```python
from build123d import *

# Parameters (mm, degrees)
ESBO_O1_W                = 36
ESBO_O1_H                = 55
RESSALTO_EXTRUS_O1_DEPTH = 75
ESBO_O2_W                = 34
ESBO_O2_H                = 30
CORTE_EXTRUS_O1_DEPTH    = 56
ESBO_O3_W                = 56
ESBO_O3_H                = 51
CORTE_EXTRUS_O2_DEPTH    = 57
ESBO_O5_R                = 5
CORTE_EXTRUS_O4_DEPTH    = 57
ESBO_O6_W                = 36
ESBO_O6_H                = 51
CORTE_EXTRUS_O5_DEPTH    = 16
ESBO_O4_R                = 5
CORTE_EXTRUS_O6_DEPTH    = 63


with BuildPart() as part:
    # Esboço1 → Ressalto-extrusão1 (new body)
    with BuildSketch(Plane.XY):
        Rectangle(ESBO_O1_W, ESBO_O1_H)
    extrude(amount=RESSALTO_EXTRUS_O1_DEPTH)

    # Esboço2 → Corte-extrusão1 (cut)
    with BuildSketch(Plane.XY.offset(75)):
        Rectangle(ESBO_O2_W, ESBO_O2_H)
    extrude(amount=-CORTE_EXTRUS_O1_DEPTH, mode=Mode.SUBTRACT)

    # Esboço3 → Corte-extrusão2 (cut)
    with BuildSketch(Plane.ZY.offset(18)):
        with Locations((47, 0)):
            Rectangle(ESBO_O3_W, ESBO_O3_H)
    extrude(amount=-CORTE_EXTRUS_O2_DEPTH, mode=Mode.SUBTRACT)

    # Esboço5 → Corte-extrusão4 (cut)
    with BuildSketch(Plane(origin=(0, 0, 0), x_dir=(-1, 0, 0), z_dir=(0, 0, -1))):
        Circle(ESBO_O5_R)
    extrude(amount=-CORTE_EXTRUS_O4_DEPTH, mode=Mode.SUBTRACT)

    # Esboço6 → Corte-extrusão5 (cut)
    with BuildSketch(Plane.XY.offset(19)):
        Rectangle(ESBO_O6_W, ESBO_O6_H)
    extrude(amount=-CORTE_EXTRUS_O5_DEPTH, mode=Mode.SUBTRACT)

    # Esboço4 → Corte-extrusão6 (cut)
    with BuildSketch(Plane.XZ.offset(27.5)):
        with Locations((0, 60)):
            Circle(ESBO_O4_R)
    extrude(amount=-CORTE_EXTRUS_O6_DEPTH, mode=Mode.SUBTRACT)


solid = part.part
```
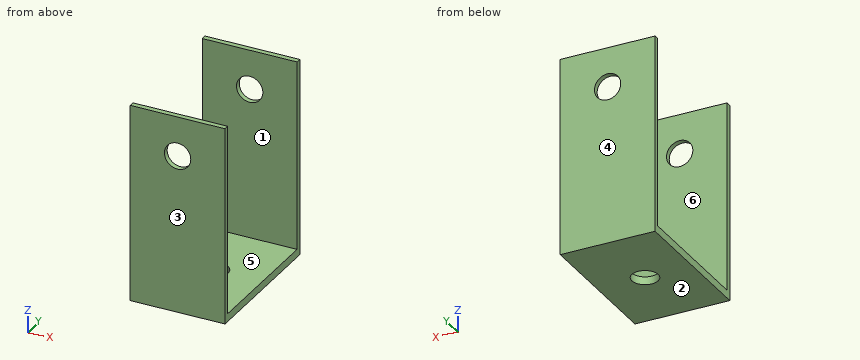
Design review of the part built by this model. Coordinates are the model's own, in mm. Face numbers are marked on the shaded views. A direction names the side the tool comes from. Give positions to 0.01 mm unless a question says otherwise; leave off trailing zeros. Loops run counter-clockwise (first coordinate to the right, second up) from the corner with the lowest first, then second, coordinate; pieces in that order, holes last. Notation, with made-up numbers: M 43,-13 L 73,-13 A13 ccw 73,6 Z; hole C 40.5,37.25 d1. An arc over 180 degrees is marked long. Return JSON: item names as keys, results as strings. Group by question number.
Item 1: Insertion check: pin 1 Ø9 at (x, y) = (0, 0) entering from +Z; pin 2 Ø2 at (x, y) = (-13, -4.5) entering from +Z. Each pin has a flat end and moves straight along its axis. Give the tip position at first contact, or say it passes through.
Item 2: We need section B-B (x = 0). Give the boundary of the cut face in (y, z).
Item 3: We need section A-A (z = 60). Give the boundary of the cut face in (x, y).
Item 4: Mouldability with a two-part tool opening along Y and no side actions: class the marked faces 3, 4, 5 and 6 as released by +Y, released by -Y, zero draft, split by the parting line, or undercut.
Item 5: Tool access review of the marked faces 1 and 2: name each direction out of +Z, -Z, +X, -X, +Y, -Y from which nothing blocks a thin tool from reaching the whole face with its end or side.
Item 6: We need section D-D (z = 26). Give the boundary of the cut face in (x, y), and give its area (3 significant figures).
Item 7: For probe 1 along Y at (x, z) = (-0.5, 32.5); probe 2 along Y at (x, z) = (0, 0.7); probe 3 along Z at (x, y) = (0, 26.2), list the stretches that pass through material, from the lowest coordinate up.
Item 8: We need section C-C (y = 0). Give the boundary of the cut face in (x, z).
Output:
{
 "1": {"pin 1": "passes through", "pin 2": "stops at z = 3"},
 "2": {"outline": "M -27.5,0 L -5,0 L -5,3 L -25.5,3 L -25.5,55 L -27.5,55 Z; M -27.5,65 L -25.5,65 L -25.5,75 L -27.5,75 Z; M 5,0 L 27.5,0 L 27.5,55 L 25.5,55 L 25.5,3 L 5,3 Z; M 25.5,65 L 27.5,65 L 27.5,75 L 25.5,75 Z"},
 "3": {"outline": "M -18,-27.5 L -5,-27.5 L -5,-25.5 L -18,-25.5 Z; M -18,25.5 L -5,25.5 L -5,27.5 L -18,27.5 Z; M 5,-27.5 L 18,-27.5 L 18,-25.5 L 5,-25.5 Z; M 5,25.5 L 18,25.5 L 18,27.5 L 5,27.5 Z"},
 "4": {"face 3": "released by -Y", "face 4": "released by +Y", "face 5": "undercut", "face 6": "undercut"},
 "5": {"face 1": "+Z, +X, -X", "face 2": "-Z, +X, -X, +Y, -Y"},
 "6": {"outline": "M -18,-27.5 L 18,-27.5 L 18,-25.5 L -18,-25.5 Z; M -18,25.5 L 18,25.5 L 18,27.5 L -18,27.5 Z", "area": "144 mm^2"},
 "7": {"probe 1": "y = -27.5 to -25.5, 25.5 to 27.5", "probe 2": "y = -27.5 to -5, 5 to 27.5", "probe 3": "z = 0 to 55, 65 to 75"},
 "8": {"outline": "M -18,0 L -5,0 L -5,3 L -18,3 Z; M 5,0 L 18,0 L 18,3 L 5,3 Z"}
}
